The model under review builds one solid part; all positions refer to its coordinate system, in mm. A direction names the side the tool comes from. Give positions to 0.01 mm unless a question says otherwise; leave off trailing zeros. Order: outer loops, then holes, each group sorted by start corner. A loop starts at its lowest first (then second) coordinate and runs counter-clockwise, first axis right, second up. Notation, with made-up numbers: (-20, -22.75) - (-10, -22.75) arc R17 ccw to (-10, -18.75) - close; hole circle Ø6 at (-20.75, -14.75). An arc over 180 degrees is marked (long way). Write item = value, one per line. Start each with the question number.
1. For P1, Ø1, axis at x = 1, z = 16, coming from the -Y side; P2, Ø2, axis at x = -3.5, z = 21, coming from the +Y side, all flat-tipped, find the tip position at first contact; note any pin that passes through.
2. Mouldability with a two-part tool opening along Y and no side actions: class faces 5 (the flat face through (-0.213, 5.523, 12.818)), 6 (the cylindrical face through (4.783, -0.938, 12.818)), 7 (the flat face through (0, -3, 26)) as pulls with the +Y half, pulls with the -Y half, needs draft (parallel to the pull), parting line crosses it, or undercut.
3. Wall thickness on probe 1 along Y at (x, z) = (1, 20.5); probe 2 along Y at (x, z) = (0.75, 5.25); probe 3 along X at (y, z) = (-0.5, 18.5): over which ranges is each line inside the solid? List them lowest first.
4. We need section A-A, the plane y = 1.5. Give the boundary of the cut face in (x, z).
5. Machinability: for faces 1 (the flat face through (3.754, 4.056, 12.818)), 2 (the flat face through (-5.023, 2.348, 12.818)), 3 (the flat face through (-4.056, 3.754, 12.818)), 4 (the flat face through (0.213, -5.523, 12.818)), which of the approach directions +Z, -Z, +X, -X, +Y, -Y give a long, thin tool a straight path to every point of the face, cutting with its end or side? Answer none if there is none.
Solid Edge part; units mm, degrees
sketch "Sketch1" plane through (0, 0, 0) normal (0, 0, 1) x (1, 0, 0)
  line L0 (4.8737, 0) -> (6.1903, 0.4329)
  arc A0 (5.9017, 1.9176) -> (6.1903, 0.4329) centre (0, 0) cw
  line L1 (5.9017, 1.9176) -> (4.5027, 1.8651)
  arc A1 (3.4462, 3.4462) -> (4.5027, 1.8651) centre (0, 0) cw
  line L2 (3.4462, 3.4462) -> (4.0711, 4.6833)
  arc A2 (2.8172, 5.529) -> (4.0711, 4.6833) centre (0, 0) cw
  line L3 (2.8172, 5.529) -> (1.8651, 4.5027)
  arc A3 (0, 4.8737) -> (1.8651, 4.5027) centre (0, 0) cw
  line L4 (0, 4.8737) -> (-0.4329, 6.1903)
  arc A4 (-1.9176, 5.9017) -> (-0.4329, 6.1903) centre (0, 0) cw
  line L5 (-1.9176, 5.9017) -> (-1.8651, 4.5027)
  arc A5 (-3.4462, 3.4462) -> (-1.8651, 4.5027) centre (0, 0) cw
  line L6 (-3.4462, 3.4462) -> (-4.6833, 4.0711)
  arc A6 (-5.529, 2.8172) -> (-4.6833, 4.0711) centre (0, 0) cw
  line L7 (-5.529, 2.8172) -> (-4.5027, 1.8651)
  arc A7 (-4.8737, 0) -> (-4.5027, 1.8651) centre (0, 0) cw
  line L8 (-4.8737, 0) -> (-6.1903, -0.4329)
  arc A8 (-5.9017, -1.9176) -> (-6.1903, -0.4329) centre (0, 0) cw
  line L9 (-5.9017, -1.9176) -> (-4.5027, -1.8651)
  arc A9 (-3.4462, -3.4462) -> (-4.5027, -1.8651) centre (0, 0) cw
  line L10 (-3.4462, -3.4462) -> (-4.0711, -4.6833)
  arc A10 (-2.8172, -5.529) -> (-4.0711, -4.6833) centre (0, 0) cw
  line L11 (-2.8172, -5.529) -> (-1.8651, -4.5027)
  arc A11 (0, -4.8737) -> (-1.8651, -4.5027) centre (0, 0) cw
  line L12 (0, -4.8737) -> (0.4329, -6.1903)
  arc A12 (1.9176, -5.9017) -> (0.4329, -6.1903) centre (0, 0) cw
  line L13 (1.9176, -5.9017) -> (1.8651, -4.5027)
  arc A13 (3.4462, -3.4462) -> (1.8651, -4.5027) centre (0, 0) cw
  line L14 (3.4462, -3.4462) -> (4.6833, -4.0711)
  arc A14 (5.529, -2.8172) -> (4.6833, -4.0711) centre (0, 0) cw
  line L15 (5.529, -2.8172) -> (4.5027, -1.8651)
  arc A15 (4.8737, 0) -> (4.5027, -1.8651) centre (0, 0) cw
extrude "Protrusion1" add sketch "Sketch1" along normal blind 26
sketch "Sketch2" plane through (0, 0, 26) normal (0, 0, 1) x (1, 0, 0)
  circle A0 centre (0, 0) radius 2.5
extrude "Cutout1" cut sketch "Sketch2" against normal through all
sketch "Sketch3" plane through (0, 0, 26) normal (0, 0, 1) x (0.95, 0.3123, 0)
  line L0 (-1.75, -1.7854) -> (-1.75, 1.7854)
  arc A0 (-1.75, -1.7854) -> (-1.75, 1.7854) centre (0, 0) cw
  line L1 (1.75, -1.7854) -> (1.75, 1.7854)
  arc A1 (1.75, 1.7854) -> (1.75, -1.7854) centre (0, 0) cw
extrude "Protrusion2" add sketch "Sketch3" against normal up to vertex (26 mm away)
properties material "ABS Plastic, high impact"
Model answer:
q1.P1 = -6.19
q1.P2 = 4.18
q2.face_5 = pulls with the +Y half
q2.face_6 = undercut
q2.face_7 = needs draft
q3.probe_1 = -6.12 to -2.29, 2.29 to 4.77
q3.probe_2 = -6.16 to -2.38, 2.38 to 4.82
q3.probe_3 = -6.19 to -1.68, 2.01 to 4.85
q4.outline = (-4.64, 0) - (-2, 0) - (-2, 26) - (-4.64, 26) - close; (1.35, 0) - (6.02, 0) - (6.02, 26) - (1.35, 26) - close
q5.face_1 = +Z, -Z, +X
q5.face_2 = +Z, -Z, -X
q5.face_3 = +Z, -Z, +Y
q5.face_4 = +Z, -Z, -Y
